Can you work these out from the model? Positions are in its coordinate system, mm. A direction names the side the tool comes from. Coordinates: 2 decimals unless noted, no trailing zeros. Use one line per item in the form item = value. Start each with the question number.
(1) Thinking about a two-plate mould opening in X: for faces 1 (the flat face through (-15, 195, 12)), 2 (the flat face through (110, 200, 12)), which applies, released by +X, released by -X, zero draft, split by the parting line, or undercut?
(2) I need wall thicknesses on line 1 (Y direction, x = 56.5, z = 19). Which ranges of the line are inside material? Lowest first, please. Write a range as [from, to].
(3) On a 3-axis mill with a long thin cutter (end or side, diameter ignored), from which of +Z, -Z, +X, -X, +Y, -Y can I reach the whole of each face in a straight line? I mean faces 3 (the flat face through (180, -190, 12)), 4 (the flat face through (-10, -200, 12)), 5 (the flat face through (-5, 195, 12)). Say none if no direction works.
(4) I'm going to push flat-ended pins straight in: pin 1 (5 mm diameter, centred on y = 197.5, z = 14, fed in from -X); pin 2 (8 mm diameter, centred on x = 78, z = 12.5, fed in from +Y); pin 3 (1 mm diameter, centred on x = 2.5, z = 15, fed in from +Y); pin 4 (5 mm diameter, centred on x = 19, z = 14, fed in from -Y). Where does each tip first touch, or does it pass through?
```python
from build123d import *

# Parameters (mm, degrees)
F1_DEPTH = 25


with BuildPart() as f1:
    # F0 (on Top) → F1 (new body)
    with BuildSketch(Plane.XY):
        Polygon((185, -200), (195, -200), (195, -190), (200, -190), (200, 190), (195, 190), (195, 200), (185, 200), (185, 190), (175, 190), (175, 200), (165, 200), (165, 190), (155, 190), (155, 200), (145, 200), (145, 190), (135, 190), (135, 200), (125, 200), (125, 190), (115, 190), (115, 200), (105, 200), (105, 190), (95, 190), (95, 200), (85, 200), (85, 190), (75, 190), (75, 200), (65, 200), (65, 190), (55, 190), (55, 200), (45, 200), (45, 190), (35, 190), (35, 200), (25, 200), (25, 190), (15, 190), (15, 200), (5, 200), (5, 190), (-5, 190), (-5, 200), (-15, 200), (-15, 190), (-25, 190), (-25, 200), (-35, 200), (-35, 190), (-45, 190), (-45, 200), (-55, 200), (-55, 190), (-65, 190), (-65, 200), (-75, 200), (-75, 190), (-85, 190), (-85, 200), (-95, 200), (-95, 190), (-105, 190), (-105, 200), (-115, 200), (-115, 190), (-125, 190), (-125, 200), (-135, 200), (-135, 190), (-145, 190), (-145, 200), (-155, 200), (-155, 190), (-165, 190), (-165, 200), (-175, 200), (-175, 190), (-185, 190), (-185, 200), (-195, 200), (-195, 190), (-200, 190), (-200, -190), (-195, -190), (-195, -200), (-185, -200), (-185, -190), (-175, -190), (-175, -200), (-165, -200), (-165, -190), (-155, -190), (-155, -200), (-145, -200), (-145, -190), (-135, -190), (-135, -200), (-125, -200), (-125, -190), (-115, -190), (-115, -200), (-105, -200), (-105, -190), (-95, -190), (-95, -200), (-85, -200), (-85, -190), (-75, -190), (-75, -200), (-65, -200), (-65, -190), (-55, -190), (-55, -200), (-45, -200), (-45, -190), (-35, -190), (-35, -200), (-25, -200), (-25, -190), (-15, -190), (-15, -200), (-5, -200), (-5, -190), (5, -190), (5, -200), (15, -200), (15, -190), (25, -190), (25, -200), (35, -200), (35, -190), (45, -190), (45, -200), (55, -200), (55, -190), (65, -190), (65, -200), (75, -200), (75, -190), (85, -190), (85, -200), (95, -200), (95, -190), (105, -190), (105, -200), (115, -200), (115, -190), (125, -190), (125, -200), (135, -200), (135, -190), (145, -190), (145, -200), (155, -200), (155, -190), (165, -190), (165, -200), (175, -200), (175, -190), (185, -190), align=None)
    extrude(amount=F1_DEPTH)


solid = f1.part
```
Worked out:
q1.face_1 = undercut
q1.face_2 = zero draft
q2.line_1 = [-190, 190]
q3.face_3 = +Z, -Z, -Y
q3.face_4 = +Z, -Z, +X, -X, -Y
q3.face_5 = +Z, -Z, +Y
q4.pin_1 = -195
q4.pin_2 = 200
q4.pin_3 = 190
q4.pin_4 = -190
